```python
from build123d import *

# Parameters (mm, degrees)
SKETCH1_R           = 1.45
SKETCH1_W           = 4.5
SKETCH1_H           = 20
BOSS_EXTRUDE1_DEPTH = 5
SKETCH2_W           = 7.5
SKETCH2_H           = 23
SKETCH2_W_2         = 4.5
SKETCH2_H_2         = 20
BOSS_EXTRUDE2_DEPTH = 5
SKETCH3_W           = 7.5
SKETCH3_H           = 23
BOSS_EXTRUDE3_DEPTH = 1
CUT_EXTRUDE1_REACH  = 33.075
SKETCH6_R           = 1.25
SKETCH7_W           = 5
SKETCH7_H           = 26
BOSS_EXTRUDE4_DEPTH = 25
SKETCH8_W           = 22.5
SKETCH8_H           = 23
BOSS_EXTRUDE5_DEPTH = 1
BOSS_EXTRUDE6_DEPTH = 23
FILLET1_R           = 0.8
BOSS_EXTRUDE7_START = -5
BOSS_EXTRUDE7_DEPTH = 5
BOSS_EXTRUDE8_START = -5
BOSS_EXTRUDE8_DEPTH = 5
SKETCH12_R          = 3.15
CUT_EXTRUDE2_DEPTH  = 3.1
FILLET2_R           = 5
BOSS_EXTRUDE9_START = -0.4
SKETCH14_R          = 1.45
BOSS_EXTRUDE9_DEPTH = 0.4


with BuildPart() as part:
    # Sketch1 → Boss-Extrude1 (new body)
    with BuildSketch(Plane.XY):
        with BuildLine():
            Line((-4.25, 0), (-4.25, 26))
            ThreePointArc((-4.25, 26), (0, 30.25), (4.25, 26))
            Line((4.25, 26), (4.25, 0))
            ThreePointArc((4.25, 0), (0, -4.25), (-4.25, 0))
        make_face()
        with Locations((0, 26)):
            Circle(SKETCH1_R, mode=Mode.SUBTRACT)
        Circle(SKETCH1_R, mode=Mode.SUBTRACT)
        with Locations((0, 13)):
            Rectangle(SKETCH1_W, SKETCH1_H, mode=Mode.SUBTRACT)
    extrude(amount=BOSS_EXTRUDE1_DEPTH)

    # Sketch2 → Boss-Extrude2 (add)
    with BuildSketch(Plane.XY.offset(5)):
        with Locations((0, 13)):
            Rectangle(SKETCH2_W, SKETCH2_H)
        with Locations((0, 13)):
            Rectangle(SKETCH2_W_2, SKETCH2_H_2, mode=Mode.SUBTRACT)
    extrude(amount=BOSS_EXTRUDE2_DEPTH)

    # Sketch3 → Boss-Extrude3 (add)
    with BuildSketch(Plane.XY.offset(10)):
        with Locations((0, 13)):
            Rectangle(SKETCH3_W, SKETCH3_H)
    extrude(amount=BOSS_EXTRUDE3_DEPTH)

    # Sketch6 → Cut-Extrude1 (cut, up to next)
    with BuildSketch(Plane.XZ.offset(-1.5), mode=Mode.PRIVATE) as cut_extrude1_sk1:
        with Locations((0, 7.153891294)):
            Circle(SKETCH6_R)
    cut_extrude1_tool1 = extrude(cut_extrude1_sk1.sketch, amount=-CUT_EXTRUDE1_REACH, mode=Mode.PRIVATE) & part.part
    add(cut_extrude1_tool1.solids().sort_by_distance((0, 1.5, 7.153891))[0], mode=Mode.SUBTRACT)

    # Sketch7 → Boss-Extrude4 (add)
    with BuildSketch(Plane.ZY.offset(4.25)):
        with Locations((2.5, 13)):
            Rectangle(SKETCH7_W, SKETCH7_H)
    extrude(amount=BOSS_EXTRUDE4_DEPTH)

    # Sketch8 → Boss-Extrude5 (add)
    with BuildSketch(Plane.XY.offset(5)):
        with Locations((-16.5, 13)):
            Rectangle(SKETCH8_W, SKETCH8_H)
    extrude(amount=BOSS_EXTRUDE5_DEPTH)

    # Sketch10 → Boss-Extrude6 (add)
    with BuildSketch(Plane.XZ.offset(-1.5)):
        Polygon((-1.5, 11), (1.5, 11), (3.75, 21), (-3.75, 21), align=None)
    extrude(amount=-BOSS_EXTRUDE6_DEPTH)

    # Fillet1
    fillet1_edges = [part.edges().sort_by_distance(p)[0] for p in [
        (-3.75, 13, 21),
        (3.75, 13, 21),
        (-3.75, 1.5, 8),
        (3.75, 1.5, 8),
        (3.75, 24.5, 8),
        (-3.75, 24.5, 8),
        (-3.75, 13, 11),
        (3.75, 13, 11),
        (-29.25, 26, 2.5),
        (-29.25, 0, 2.5),
    ]]
    fillet(fillet1_edges, radius=FILLET1_R)

    # Sketch11 → Boss-Extrude7 (add)
    with BuildSketch(Plane.XY.offset(5).offset(BOSS_EXTRUDE7_START)):
        with BuildLine():
            Line((-4.25, 0), (-4.25, -11.262558254))
            Line((-4.25, -11.262558254), (4.25, -11.262558254))
            Line((4.25, -11.262558254), (4.25, 0))
            ThreePointArc((4.25, 0), (0, -4.25), (-4.25, 0))
        make_face()
    extrude(amount=BOSS_EXTRUDE7_DEPTH)

    # Sketch13 → Boss-Extrude8 (add)
    with BuildSketch(Plane.XY.offset(5).offset(BOSS_EXTRUDE8_START)):
        with BuildLine():
            Line((4.25, -11.262558254), (5.75, -11.262558254))
            Line((5.75, -11.262558254), (5.75, 30.25))
            Line((5.75, 30.25), (0, 30.25))
            ThreePointArc((0, 30.25), (3.00520382, 29.00520382), (4.25, 26))
            Line((4.25, 26), (4.25, -11.262558254))
        make_face()
    extrude(amount=BOSS_EXTRUDE8_DEPTH)

    # Sketch12 → Cut-Extrude2 (cut)
    with BuildSketch(Plane(origin=(0, 0, 0), x_dir=(-1, 0, 0), z_dir=(0, 0, -1))):
        with Locations((-1.6, -6.45)):
            Circle(SKETCH12_R)
    extrude(amount=-CUT_EXTRUDE2_DEPTH, mode=Mode.SUBTRACT)

    # Fillet2
    fillet2_edges = [part.edges().sort_by_distance(p)[0] for p in [
        (5.75, 30.25, 2.5),
        (5.75, -11.262558254, 2.5),
        (-4.25, -11.262558254, 2.5),
    ]]
    fillet(fillet2_edges, radius=FILLET2_R - 0.0001)  # a hair under: the kernel refuses the full size

    # Sketch14 → Boss-Extrude9 (add)
    with BuildSketch(Plane.XY.offset(5).offset(BOSS_EXTRUDE9_START)):
        with Locations((0, 26)):
            Circle(SKETCH14_R)
        Circle(SKETCH14_R)
    extrude(amount=BOSS_EXTRUDE9_DEPTH)


solid = part.part
```
The model under review builds one solid part; all positions refer to its coordinate system, in mm. A direction names the side the tool comes from. Round coordinates to 2 decimals unless told otherwise and drop trailing zeros. Write each loop counter-clockwise with the first axis right and the second up, starting at its lowest first coordinate (ties: lowest second). Pieces come first, ordered by that corner, then holes.
(1) Machinability: for faces 1 (the cylindrical face through (2.01, -3.327, 1.528)), 2 (the flat face through (-4.25, -3, 2)), 3 (the flat face through (2, 13, 11)), 4 (the flat face through (-5.25, 12.8, 5.5)), which of the approach directions +Z, -Z, +X, -X, +Y, -Y give a long, thin tool a straight path to every point of the face, cutting with its end or side? Answer none if there is none.
(2) Mouldability with a two-part tool opening along Z and no side actions: class faces 5 (the flat face through (-16.7, 1.5, 5.5)), 6 (the flat face through (-2, 13, 11)), 7 (the flat face through (-17, 13, 6)), 8 (the flat face through (0, 26, 4.6)) as +Z half, -Z half, draft (parallel to the pull), parting line (faces both ways), or undercut.
(3) We need section A-A on y = 14. Give the boundary of the cut face in (x, z).
(4) We need section B-B on z = 1.5. Give the number of separate pieces and of enclosed holes in the cut face, and give its area (4 significant figures).
(5) We need section C-C on x = -10.5. Give the boundary of the cut face in (y, z), and give its area (3 significant figures).
(6) We need section D-D on y = -7.5. Give the boundary of the cut face in (x, z).
(7) Wall thickness on L1, parallel to X at y = 11, z = 1.5; L2, parallel to Y at x = 1.6, z = 1.3; L3, parallel to Z at x = 0, y = 2.65: over which ranges is each line inside the solid? List them lowest first.
(8) Insertion check: pin 1 (4.5 mm diameter, centred on x = 0, y = 26, fed in from -Z); pin 2 (4 mm diameter, centred on y = 11, z = 11, fed in from -X); pin 3 (1.1 mm diameter, centred on x = -16.5, z = 5.5, fed in from -Y); pin 4 (3 mm diameter, centred on x = 0, z = 7.15, fed in from -Y). Each pin has a flat end and moves straight along its axis. Give the tip position at first contact, or say it passes through.
Findings below:
1. face 1: -Z
1. face 2: +Z, -Z, -X, -Y
1. face 3: +X, +Y, -Y
1. face 4: +Z, +Y, -Y
2. face 5: draft
2. face 6: undercut
2. face 7: +Z half
2. face 8: -Z half
3. outline: (-29.25, 0) - (-2.25, 0) - (-2.25, 10) - (2.25, 10) - (2.25, 0) - (5.75, 0) - (5.75, 5) - (3.75, 5) - (3.75, 10.2) arc R0.8 ccw to (2.95, 11) - (1.5, 11) - (3.53, 20.02) arc R0.8 ccw to (2.75, 21) - (-2.75, 21) arc R0.8 ccw to (-3.53, 20.02) - (-1.5, 11) - (-2.95, 11) arc R0.8 ccw to (-3.75, 10.2) - (-3.75, 5) - (-5.25, 5) - (-5.25, 6) - (-27.75, 6) - (-27.75, 5) - (-29.25, 5) - close
4. separate pieces: 1
4. enclosed holes: 4
4. area: 910.5 mm2
5. outline: (0, 0) - (26, 0) - (26, 5) - (24.5, 5) - (24.5, 6) - (1.5, 6) - (1.5, 5) - (0, 5) - close
5. area: 153 mm2
6. outline: (-4.09, 0) - (-1.37, 0) - (-1.37, 3.1) - (4.57, 3.1) - (4.57, 0) - (5.59, 0) - (5.59, 5) - (-4.09, 5) - close
7. L1: x = -29.25 to -2.25, 2.25 to 5.75
7. L2: y = -11.19 to -9.6, -3.3 to 3, 23 to 30.18
7. L3: z = 0 to 5.9, 8.4 to 21
8. pin 1: stops at z = 0
8. pin 2: stops at x = -3.75
8. pin 3: stops at y = 0
8. pin 4: stops at y = 1.5
